Autodesk Inventor part; units mm, degrees
ref_plane "XZ Plane" through (0, 0, 0) normal (0, 1, 0) x (-1, 0, 0)
ref_plane "XY Plane" through (0, 0, 0) normal (0, 0, 1) x (1, 0, 0)
sketch "Sketch1" plane through (0, 0, 0) normal (0, 1, 0) x (-1, 0, 0)
  circle A0 centre (0, 0) radius 1.1
  circle A1 centre (0, 0) radius 2.575
  dimension "d0" = 2.2
  dimension "d1" = 5.15
extrude "Extrusion1" add sketch "Sketch1" along normal blind 18
sketch "Sketch2" plane through (0, 0, 0) normal (0, 0, 1) x (1, 0, 0)
  line L0 (2.575, 18) -> (-2.575, 18)
  line L1 (2.575, 0) -> (-2.575, 0)
  line L2 (-2.575, 0) -> (-2.575, 18)
  line L3 (-2.575, 16) -> (2.5173, 16)
  line L4 (2.575, 18) -> (-2.575, 18)
  line L5 (0, 18) -> (0, 0)
  circle A0 centre (0, 13.9) radius 2.1
  line L6 (-2.1, 13.9) -> (2.1, 13.9)
  line L7 (2.1, 13.9) -> (2.1, 18)
  line L8 (2.1, 18) -> (-2.1, 18)
  line L9 (-2.1, 18) -> (-2.1, 13.9)
  point P0 (2.1, 16)
  point P1 (-2.1, 16)
  point P2 (0, 16)
  dimension "d5" = 4.2
  dimension "d4" = 2
extrude "Extrusion2" cut sketch "Sketch2" along normal blind 12 contours L7 L3 L5 L0 | L5 L3 L9 L0 | L7 A0 L3 | A0 L9 L3 | A0 L6 L5 | L5 L6 A0 | A0 L5 L6 | L5 A0 L6
sketch "Sketch3" plane through (0, 0, 0) normal (1, 0, 0) x (0, 1, 0)
  line L0 (0, -2.575) -> (0, 2.575)
  line L1 (0, 2.575) -> (11.8, 2.575)
  line L2 (16, 2.575) -> (16, -2.525)
  line L3 (18, 1.1) -> (18, -1.1)
  line L4 (18, 0) -> (0, 0)
  circle A0 centre (13.9, 0) radius 2.1
  line L5 (13.9, 1.4902) -> (18, 1.4902)
  line L6 (18, 1.4902) -> (13.9, 1.4902)
  line L7 (13.9, 2.1) -> (18, 2.1)
  line L8 (18, 2.1) -> (18, -2.1)
  line L9 (18, -2.1) -> (13.9, -2.1)
  line L10 (13.9, -2.1) -> (13.9, 2.1)
  point P0 (18, -2.575)
  point P1 (18, 2.575)
  dimension "d9" = 4.2
  dimension "d8" = 2
extrude "Extrusion3" cut sketch "Sketch3" along normal up to next
properties part number "motor_shaft_adapter"
Design review of the part built by this model. Coordinates are the model's own, in mm. A direction names the side the tool comes from. Coordinates: 2 decimals unless noted, no trailing zeros. Order: outer loops, then holes, each group sorted by start corner. A loop starts at its lowest first (then second) coordinate and runs counter-clockwise, first axis right, second up. Notation, with made-up numbers: (56, 20) - (71, 20) arc R14 cw to (71, 30) - close; hole circle Ø4 at (-0.5, 47). An arc over 180 degrees is marked (long way). Put each result on its own line as item: value.
1) Take a section at C-C, the plane y = 15.25. Give the boundary of the cut face in (x, z) (3 decimals), and give its area (3 significant figures).
Response values:
outline: (-2.1, 0) - (-2.1, 1.49) arc R2.575 ccw to (1.49, -2.1) - (0, -2.1) - (0, -1.1) arc R1.1 cw to (-1.1, 0) - close
area: 5.22 mm²
2) The part is to be moulded in two halves that separate along Z. For faces 1 (the face through (-2.456, 6.874, -0.773)), 2 (the face through (1.27, 12.13, -1.13)), 3 (the face through (1, 16, -2.1)), say which applies: released by +Z, released by -Z, zero draft, split by the parting line, or undercut.
Response values:
face 1: split by the parting line
face 2: undercut
face 3: released by +Z
3) Take a section at B-B, the plane z = 0.6. Give the boundary of the cut face in (x, y).
Response values:
outline: (-2.5, 0) - (-0.92, 0) - (-0.92, 12.01) arc R2.1 cw to (-2.1, 13.9) - (-2.1, 18) - (-2.5, 18) - close; (0.92, 0) - (2.5, 0) - (2.5, 11.89) - (0.92, 11.89) - close
4) Insertion check: P1, Ø0.8, axis at x = -1.5, y = 15.5, coming from the +Z side; P2, Ø1.2, axis at x = 1, y = 16.5, coming from the +Z side; P3, Ø2, axis at y = 9.5, z = 2, coming from the +X side; P4, Ø2, axis at x = 0, z = 0, coming from the +Y side. Each pin has a flat end and moves straight along its axis. Give the tip position at first contact, or say it passes through.
Response values:
P1: stops at z = 0
P2: stops at z = -2.1
P3: stops at x = 2.37
P4: passes through
5) Tool access review of faces 4 (the face through (0, 15, -1.6)), 5 (the face through (-1, 0, -1)), 6 (the face through (-1.068, 12.092, 1.27)): name each direction out of +Z, -Z, +X, -X, +Y, -Y from which nothing blocks a thin tool from reaching the whole face with its end or side.
Response values:
face 4: +Z, +X, +Y
face 5: +Z, -Z, +X, -X, -Y
face 6: +Z, +Y
6) Wall thickness on L1, parallel to Z at x = 0, y = 8.5 (3 decimals); L2, parallel to X at y = 12, z = 0 (3 decimals): over which ranges is each line inside the solid? List them lowest first. Write a range as from..to.
Response values:
L1: z = -2.575..-1.1, 1.1..2.575
L2: x = -2.575..-1.1
7) Take a section at D-D, the plane y = 2.75. Give the boundary of the cut face in (x, z) (3 decimals).
Response values:
outline: circle Ø5.15 at (0, 0); hole circle Ø2.2 at (0, 0)
8) Take a section at A-A, the plane x = -0.7. Give the boundary of the cut face in (y, z).
Response values:
outline: (0, -2.48) - (18, -2.48) - (18, -0.85) - (0, -0.85) - close; (0, 0.85) - (11.92, 0.85) - (11.92, 2.48) - (0, 2.48) - close
